The model under review builds one solid part; all positions refer to its coordinate system, in mm. Face numbers are marked on the shaded views. Round coordinates to 2 decimals unless told otherwise and drop trailing zeros. Loops run counter-clockwise (first coordinate to the right, second up) from the corner with the lowest first, then second, coordinate; pieces in that order, holes last. Notation, with made-up numbers: M 53.25,-26 L 98.25,-26 A14 cw 98.25,-5 Z; hole C 89.5,-17.75 d7. An arc over 180 degrees is marked long. One line per question, with ' | ' between items.
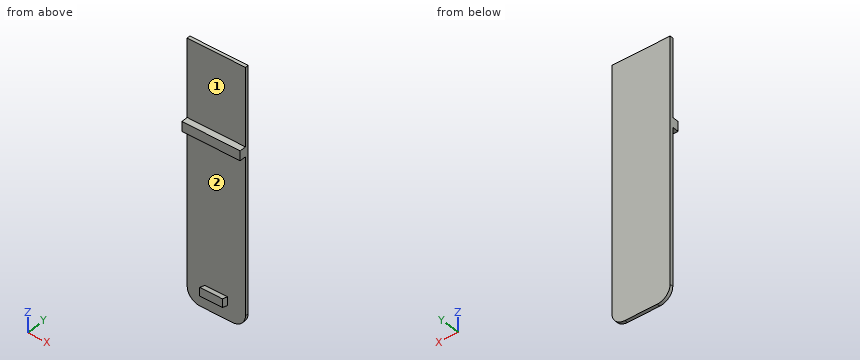
from build123d import *

# Parameters (mm, degrees)
SKETCH1_W           = 18
SKETCH1_H           = 55
BOSS_EXTRUDE1_DEPTH = 1
SKETCH2_W           = 18
SKETCH2_H           = 3
BOSS_EXTRUDE2_DEPTH = 2
SKETCH3_W           = 18
SKETCH3_H           = 1
BOSS_EXTRUDE3_DEPTH = 24
SKETCH4_W           = 7
SKETCH4_H           = 2
BOSS_EXTRUDE4_DEPTH = 2
FILLET1_R           = 4
BOSS_EXTRUDE5_DEPTH = 7


with BuildPart() as part:
    # Sketch1 → Boss-Extrude1 (new body)
    with BuildSketch(Plane(origin=(0, 0, 0), x_dir=(1, 0, 0), z_dir=(0, 1, 0))):
        with Locations((9, -27.5)):
            Rectangle(SKETCH1_W, SKETCH1_H)
    extrude(amount=BOSS_EXTRUDE1_DEPTH)

    # Sketch2 → Boss-Extrude2 (add)
    with BuildSketch(Plane.XZ):
        with Locations((9, 53.5)):
            Rectangle(SKETCH2_W, SKETCH2_H)
    extrude(amount=BOSS_EXTRUDE2_DEPTH)

    # Sketch3 → Boss-Extrude3 (add)
    with BuildSketch(Plane.XY.offset(55)):
        with Locations((9, 0.5)):
            Rectangle(SKETCH3_W, SKETCH3_H)
    extrude(amount=BOSS_EXTRUDE3_DEPTH)

    # Sketch4 → Boss-Extrude4 (add)
    with BuildSketch(Plane.XZ):
        with Locations((9, 6)):
            Rectangle(SKETCH4_W, SKETCH4_H)
    extrude(amount=BOSS_EXTRUDE4_DEPTH)

    # Fillet1
    fillet1_edges = [part.edges().sort_by_distance(p)[0] for p in [
        (0, 0.5, 0),
        (18, 0.5, 0),
    ]]
    fillet(fillet1_edges, radius=FILLET1_R)

    # Sketch5 → Boss-Extrude5 (add)
    with BuildSketch(Plane.ZY.offset(-5.5)):
        Polygon((7, 0), (7.615831877, -2), (7, -2), align=None)
        Polygon((5, 0), (5, -2), (4.384168123, 0), align=None)
    extrude(amount=-BOSS_EXTRUDE5_DEPTH)


solid = part.part
1) Add section A-A on x = 9.5. State the section outline as (y, z) points, then the cut area to 3 significant figures.
Output values:
outline: M -2,5 L 0,4.38 L 0,0 L 1,0 L 1,79 L 0,79 L 0,55 L -2,55 L -2,52 L 0,52 L 0,7 L -2,7.62 Z | area: 90.2 mm²
2) Add section C-C on z = 72.5. State the section outline as (x, y) points.
Output values:
outline: M 0,0 L 18,0 L 18,1 L 0,1 Z
3) For line 1 (Y direction, x = 13.25, z = 28); line 2 (Z direction, x = 1.5, y = -1.7); line 3 (Z direction, x = 9.5, y = -0.2), list the stretches that pass through material, from the lowest coordinate up.
Output values:
line 1: y = 0 to 1 | line 2: z = 52 to 55 | line 3: z = 4.45 to 7.06, 52 to 55
4) Add section D-D on x = 15.75. State the section outline as (y, z) points.
Output values:
outline: M -2,52 L 0,52 L 0,0.4 L 1,0.4 L 1,79 L 0,79 L 0,55 L -2,55 Z
5) Add section B-B on y = -0.6. State the section outline as (x, z) points, then the cut area to 3 significant figures.
Output values:
outline: M 0,52 L 18,52 L 18,55 L 0,55 Z; M 5.5,4.57 L 12.5,4.57 L 12.5,7.18 L 5.5,7.18 Z | area: 72.3 mm²
6) Insertion check: P1, Ø5.5, axis at x = 11.5, z = 72.5, coming from the -Y side; P2, Ø1, axis at y = -1.5, z = 6, coming from the -X side; P3, Ø1.5, axis at x = 10.5, y = -1.5, coming from the -Z side. Each pin has a flat end and moves straight along its axis. Give the tip position at first contact, or say it passes through.
Output values:
P1: stops at y = 0 | P2: stops at x = 5.5 | P3: stops at z = 4.62
7) Mouldability with a two-part tool opening along Z and no side actions: class the marked faces 1 and 2 as +Z half, -Z half, draft (parallel to the pull), parting line (faces both ways), or undercut.
Output values:
face 1: draft | face 2: undercut
